Geometry: final body of the model. Coordinates: model frame, mm. Face numbers are marked on the shaded views. A direction names the side the tool comes from. Give positions to 0.01 mm unless a question says otherwise; leave off trailing zeros. Order: outer loops, then holes, each group sorted by start corner. A loop starts at its lowest first (then second) coordinate and runs counter-clockwise, first axis right, second up. Notation, with made-up numbers: (-19, -31.5) - (-5, -31.5) arc R25 cw to (-5, -18.5) - close; hole circle Ø10 at (-17.5, 27). An arc over 180 degrees is marked (long way). Write item = value, one per line. Start each with the question number.
from build123d import *

# Parameters (mm, degrees)
BOSS_EXTRUDE1_DEPTH = 20
BOSS_EXTRUDE3_DEPTH = 4
SKETCH11_W          = 8
SKETCH11_H          = 4.067153682
BOSS_EXTRUDE8_DEPTH = 1
BOSS_EXTRUDE7_DEPTH = 20
FILLET1_R           = 2


with BuildPart() as part:
    # Sketch1 → Boss-Extrude1 (new body)
    with BuildSketch(Plane(origin=(0, 0, 0), x_dir=(1, 0, 0), z_dir=(0, 1, 0))):
        Polygon((7.95, 0), (7.95, -2.04), (4.048, -6.152414984), (-4.048, -6.152414984), (-7.95, -2.04), (-7.95, 0), align=None)
    extrude(amount=-BOSS_EXTRUDE1_DEPTH)

    # Sketch4 → Boss-Extrude3 (add, symmetric)
    with BuildSketch(Plane(origin=(0, 0, 0), x_dir=(0, 0, -1), z_dir=(1, 0, 0))):
        Polygon((13.481068451, 0), (0, 0), (0, -12.539693486), (17.27808352, -1.457537526), align=None)
    extrude(amount=BOSS_EXTRUDE3_DEPTH, both=True)

    # Sketch11 → Boss-Extrude8 (add)
    with BuildSketch(Plane(origin=(0, 4.510297753, -1.731341095), x_dir=(1, 0, 0), z_dir=(0, 0.933580426, -0.35836795))):
        with Locations((0, 14.619238475)):
            Rectangle(SKETCH11_W, SKETCH11_H)
    extrude(amount=BOSS_EXTRUDE8_DEPTH)

    # Sketch10 → Boss-Extrude7 (add)
    with BuildSketch(Plane(origin=(0, -4.510297753, -11.749727356), x_dir=(1, 0, 0), z_dir=(0, 0.35836795, 0.933580426))):
        Polygon((-7.95, 4.831182858), (-7.95, 6.871182858), (-4.048, 10.983597842), (4.048, 10.983597842), (7.95, 6.871182858), (7.95, 4.831182858), align=None)
    extrude(amount=-BOSS_EXTRUDE7_DEPTH)

    # Fillet1
    fillet1_edges = [part.edges().sort_by_distance(p)[0] for p in [
        (0, -12.539693486, 0),
        (0, -1.457537526, -17.27808352),
        (0, 0, -13.481068451),
    ]]
    fillet(fillet1_edges, radius=FILLET1_R)


solid = part.part
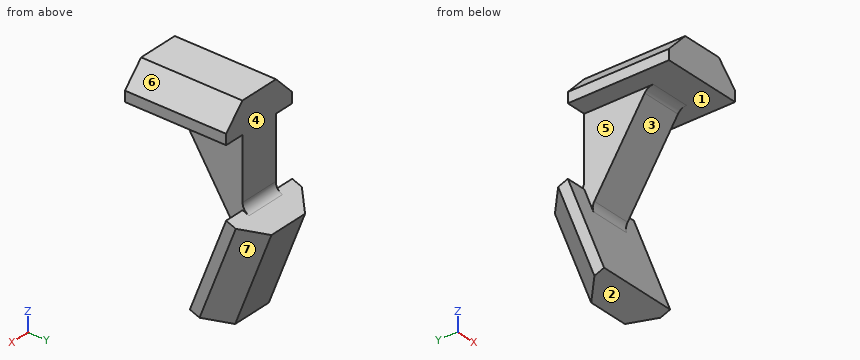
Q1. Set-up query: the marked faces 1, 2, 3 and 4. Return all of +Z, -Z, +X, -X, +Y, -Y with unobstructed straight access to the full face (end or side cutting, diameter ignored); none if empty.
Q2. Section B-B, the plane x = 6. Return the cut outline in (y, z), then the cut area to 3 significant figures.
Q3. Section D-D, the plane z = -30.5. Return the cut outline in (x, y).
Q4. Material intervals for line 1 along Y through (x, z) = (-2, 1.5); line 2 along X through (y, z) = (-1.5, -10); line 3 along Z through (x, y) = (0.5, -16), sorted ascending. Write a range as from..to.
Q5. Pull-direction query (Z, two-part tool) for the marked faces 5, 6 and 7; classes: +Z half, -Z half, draft (parallel to the pull), parting line (faces both ways), or undercut.
Q6. Contact query for flat-ended pins moving along their axis: pin 1 (1 mm diameter, centred on x = -0.5, z = -12, fed in from -Y); pin 2 (5 mm diameter, centred on x = 4, z = -19.5, fed in from -Y); pin 3 (4 mm diameter, centred on x = 1, z = -6, fed in from -Y). Output: stop coordinate, or through.
Q7. Section A-A, the plane y = -6.5. Return the cut outline in (x, z).
Q8. Section C-C, the plane y = -9.5. Return the cut outline in (x, z).
The answers:
q1.face_1 = -Y
q1.face_2 = -Z, +X, -X, -Y
q1.face_3 = +X, -X, -Y
q1.face_4 = +Z, +X, -X, +Y
q2.outline = (-20, 0) - (0, 0) - (0, 4.1) - (-20, 4.1) - close; (-7.17, -32.15) - (-3.34, -33.62) - (3.82, -14.95) - (0, -13.48) - close
q2.area = 164 mm²
q3.outline = (-7.95, -6.53) - (7.95, -6.53) - (7.95, -4.35) - (4.05, 0.06) - (-4.05, 0.06) - (-7.95, -4.35) - close
q4.line_1 = -20..0
q4.line_2 = -4..4
q4.line_3 = 0..6.15
q5.face_5 = undercut
q5.face_6 = +Z half
q5.face_7 = -Z half
q6.pin_1 = -5.16
q6.pin_2 = -3.27
q6.pin_3 = -9.97
q7.outline = (-7.95, -32.41) - (7.95, -32.41) - (7.95, -30.41) - (-7.95, -30.41) - close; (-7.95, 0) - (-4, 0) - (-4, -9.42) - (4, -9.42) - (4, 0) - (7.95, 0) - (7.95, 2.04) - (4.05, 6.15) - (-4.05, 6.15) - (-7.95, 2.04) - close
q8.outline = (-7.95, 0) - (-4, 0) - (-4, -4.74) - (4, -4.74) - (4, 0) - (7.95, 0) - (7.95, 2.04) - (4.05, 6.15) - (-4.05, 6.15) - (-7.95, 2.04) - close
